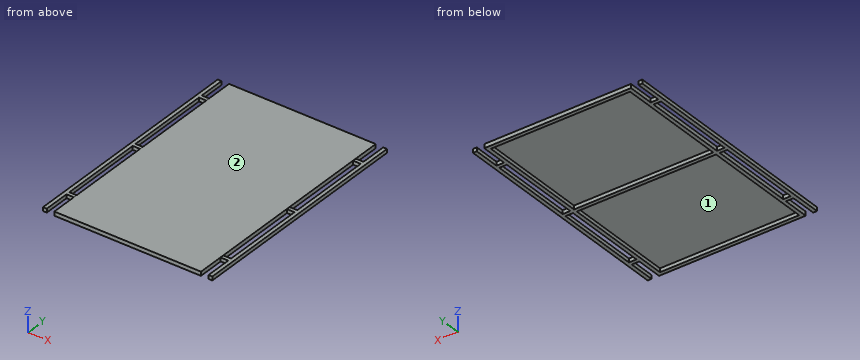
from build123d import *

# Parameters (mm, degrees)
F0_W      = 990.6
F0_H      = 1574.8
F1_DEPTH  = 1.5875
F2_W      = 990.6
F2_H      = 1574.8
F2_W_2    = 939.8
F2_H_2    = 749.3
F3_DEPTH  = 25.4
F4_W      = 25.4
F4_H      = 25.4
F5_DEPTH  = 50.8
F6_W      = 25.4
F6_H      = 25.4
F7_DEPTH  = 1574.8
F8_W      = 25.4
F8_H      = 25.4
F9_DEPTH  = 50.8
F10_W     = 25.4
F10_H     = 25.4
F11_DEPTH = 1574.8


with BuildPart() as f1:
    # F0 (on Top) → F1 (new body)
    with BuildSketch(Plane.XY):
        with Locations((495.3, -787.4)):
            Rectangle(F0_W, F0_H)
    extrude(amount=F1_DEPTH)

    # F2 (on face) → F3 (join)
    with BuildSketch(Plane(origin=(0, 0, 0), x_dir=(1, 0, 0), z_dir=(0, 0, -1))):
        with Locations((495.3, 787.4)):
            Rectangle(F2_W, F2_H)
        with Locations((495.3, 400.05)):
            Rectangle(F2_W_2, F2_H_2, mode=Mode.SUBTRACT)
        with Locations((495.3, 1174.75)):
            Rectangle(F2_W_2, F2_H_2, mode=Mode.SUBTRACT)
    extrude(amount=F3_DEPTH)

    # F4 (on face) → F5 (join)
    with BuildSketch(Plane(origin=(0, 0, 0), x_dir=(0, -1, 0), z_dir=(-1, 0, 0))):
        with Locations((190.5, -12.7)):
            Rectangle(F4_W, F4_H)
        with Locations((787.4, -12.7)):
            Rectangle(F4_W, F4_H)
        with Locations((1384.3, -12.7)):
            Rectangle(F4_W, F4_H)
    extrude(amount=F5_DEPTH)

    # F6 (on face) → F7 (join)
    with BuildSketch(Plane(origin=(0, 0, 0), x_dir=(-1, 0, 0), z_dir=(0, 1, 0))):
        with Locations((63.5, -12.7)):
            Rectangle(F6_W, F6_H)
    extrude(amount=-F7_DEPTH)

    # F8 (on face) → F9 (join)
    with BuildSketch(Plane.YZ.offset(990.6)):
        with Locations((-1384.3, -12.7)):
            Rectangle(F8_W, F8_H)
        with Locations((-787.4, -12.7)):
            Rectangle(F8_W, F8_H)
        with Locations((-190.5, -12.7)):
            Rectangle(F8_W, F8_H)
    extrude(amount=F9_DEPTH)

    # F10 (on face) → F11 (join)
    with BuildSketch(Plane(origin=(0, 0, 0), x_dir=(-1, 0, 0), z_dir=(0, 1, 0))):
        with Locations((-1054.1, -12.7)):
            Rectangle(F10_W, F10_H)
    extrude(amount=-F11_DEPTH)


solid = f1.part
Geometry: final body of the model. Coordinates: model frame, mm. Face numbers are marked on the shaded views. Give positions to 0.01 mm unless a question says otherwise; leave off trailing zeros. Loops run counter-clockwise (first coordinate to the right, second up) from the corner with the lowest first, then second, coordinate; pieces in that order, holes last. Notation, with made-up numbers: M 8,36 L 15,36 A19 cw 15,68 Z; hole C 3.25,51 d4. An arc over 180 degrees is marked long. Put each result on its own line as item: value. Start each with the question number.
1) Cut plane C-C (z = -16.5). Give the number of separate pieces and of enclosed holes in the cut face, then the cut area to 3 significant figures.
2) Ray query, line 1 along Y through (x, z) = (-26, -11.5); line 2 along Y through (x, z) = (886.5, -1.25); line 3 along X through (y, z) = (-893, -17). Return the intervals inside material, ascending.
3) Contact query for flat-ended pins moving along their axis: pin 1 (12.5 mm diameter, centred on x = -17, z = -13, fed in from +Y); pin 2 (1.5 mm diameter, centred on x = 275.5, y = -703.5, fed in from -Z); pin 3 (7.5 mm diameter, centred on x = -21.5, z = -10, fed in from -Y). Output: stop coordinate, or through.
4) Cut plane B-B (x = 222.5). Output: boundary loops of the cut face in (y, z), then the cut area to 3 significant figures.
5) Pull-direction query (Y, two-part tool) for the marked faces 1 and 2; classes: pulls with the +Y half, pulls with the -Y half, needs draft (parallel to the pull), parting line crosses it, or undercut.
6) Cut plane A-A (y = -330). Output: boundary loops of the cut face in (x, z).
Verdict:
1. separate pieces: 1
1. enclosed holes: 6
1. area: 239,000 mm2
2. line 1: -1397 to -1371.6, -800.1 to -774.7, -203.2 to -177.8
2. line 2: -1574.8 to -1549.4, -800.1 to -774.7, -25.4 to 0
2. line 3: -76.2 to -50.8, 0 to 25.4, 965.2 to 990.6, 1041.4 to 1066.8
3. pin 1: y = -177.8
3. pin 2: z = 0
3. pin 3: y = -1397
4. outline: M -1574.8,-25.4 L -1549.4,-25.4 L -1549.4,0 L -800.1,0 L -800.1,-25.4 L -774.7,-25.4 L -774.7,0 L -25.4,0 L -25.4,-25.4 L 0,-25.4 L 0,1.59 L -1574.8,1.59 Z
4. area: 4,440 mm2
5. face 1: undercut
5. face 2: needs draft
6. outline: M -76.2,-25.4 L -50.8,-25.4 L -50.8,0 L -76.2,0 Z; M 0,-25.4 L 25.4,-25.4 L 25.4,0 L 965.2,0 L 965.2,-25.4 L 990.6,-25.4 L 990.6,1.59 L 0,1.59 Z; M 1041.4,-25.4 L 1066.8,-25.4 L 1066.8,0 L 1041.4,0 Z
